from build123d import *

# Parameters (mm, degrees)
PAD002_DEPTH           = 18
CHAMFER001_SIZE        = 1
SKETCH004_W            = 20
SKETCH004_H            = 20
POCKET001_DEPTH        = 2
LINEARPATTERN001_COUNT = 3
LINEARPATTERN001_PITCH = 4
PAD003_DEPTH           = 6
CHAMFER002_SIZE        = 1


with BuildPart() as part:
    # Sketch003 → Pad002 (new body)
    with BuildSketch(Plane.XY):
        with BuildLine():
            ThreePointArc((8, 5.030159), (-9.45, 0), (8, -5.030159))
            Line((8, 5.030159), (8, -5.030159))
        make_face()
    extrude(amount=PAD002_DEPTH)

    # Chamfer001
    chamfer001_edges = [part.edges().sort_by_distance(p)[0] for p in [
        (-9.45, 0, 18),
        (8, 0, 18),
    ]]
    chamfer(chamfer001_edges, length=CHAMFER001_SIZE)

    # Sketch004 → Pocket001 (cut)
    with BuildSketch(Plane.XY.offset(3)):
        with Locations((12.12132, -12.12132)):
            Rectangle(SKETCH004_W, SKETCH004_H)
        with Locations((12.12132, 12.12132)):
            Rectangle(SKETCH004_W, SKETCH004_H)
        with Locations((-12.12132, 12.12132)):
            Rectangle(SKETCH004_W, SKETCH004_H)
        with Locations((-12.12132, -12.12132)):
            Rectangle(SKETCH004_W, SKETCH004_H)
    pocket001 = extrude(amount=POCKET001_DEPTH, mode=Mode.SUBTRACT)

    # LinearPattern001: Pocket001 ×3
    with Locations(*[(0, 0, i * LINEARPATTERN001_PITCH) for i in range(1, LINEARPATTERN001_COUNT)]):
        add(pocket001, mode=Mode.SUBTRACT)

    # Sketch005 → Pad003 (join)
    with BuildSketch(Plane.XY):
        Polygon((-12, 9), (-12, -13), (-11, -14), (7, -14), (8, -13), (8, 9), (7, 10), (-11, 10), align=None)
    extrude(amount=-PAD003_DEPTH)

    # Chamfer002
    chamfer002_edges = [part.edges().sort_by_distance(p)[0] for p in [
        (-2, 10, -6),
        (-11.5, 9.5, -6),
        (-12, -2, -6),
        (-11.5, -13.5, -6),
        (-2, -14, -6),
        (7.5, -13.5, -6),
        (8, -2, -6),
        (7.5, 9.5, -6),
    ]]
    chamfer(chamfer002_edges, length=CHAMFER002_SIZE)


solid = part.part
The listing builds one solid part. Answer for the finished solid, in the listing's coordinates (mm). A direction names the side the tool comes from. Give positions to 0.01 mm unless a question says otherwise; leave off trailing zeros. Write each loop counter-clockwise with the first axis right and the second up, starting at its lowest first coordinate (ties: lowest second). Pieces come first, ordered by that corner, then holes.
1) Section A-A (y = 0) is taken. Write down the section's boundary in (x, z), and give its area (3 significant figures).
2) Section B-B (x = 0) is taken. Write down the section's boundary in (y, z).
3) Find the intervals of material crossed by L1, parallel to Z at x = 3.5, y = 6; L2, parallel to Z at x = 7.25, y = -5.75; L3, parallel to Z at x = -1, y = -11.75, in increasing order.
4) For a pull along Z with two mould halves and no side action, classify faces 1 (the face through (-2, -2, -6)), 2 (the face through (-5, -5, 11)), 3 (the face through (-12, -2, -2)) as pulls with the +Z half, pulls with the -Z half, needs draft (parallel to the pull), parting line crosses it, or undercut.
5) Given P1, Ø12, axis at x = 4.5, z = 15, coming from the -Y side; P2, Ø2, axis at y = -6.5, z = 11.5, coming from the -X side; P3, Ø1, axis at x = -6.5, z = 12, coming from the -Y side, each flat-ended and moving along its own axis, determine where each tip first touches the part or whether it passes through.
6) A tool of negligible diameter and unlimited length cuts with its end or side. For faces 4 (the face through (4, -5, 7)), 5 (the face through (5, 2.121, 4)), 6 (the face through (-6, -2.121, 4)), from which of +Z, -Z, +X, -X, +Y, -Y can it reach the whole face along a straight path? Write none if from no direction.
7) Section C-C (z = 14.5) is taken. Write down the section's boundary in (x, y).
Response:
1. outline: (-12, -5) - (-11, -6) - (7, -6) - (8, -5) - (8, 17) - (7, 18) - (-8.45, 18) - (-9.45, 17) - (-9.45, 0) - (-12, 0) - close
1. area: 432 mm2
2. outline: (-14, -5) - (-13, -6) - (9, -6) - (10, -5) - (10, 0) - (9.45, 0) - (9.45, 17) - (8.45, 18) - (-8.45, 18) - (-9.45, 17) - (-9.45, 0) - (-14, 0) - close
3. L1: z = -6 to 3, 5 to 7, 9 to 11, 13 to 18
3. L2: z = -5.75 to 3, 5 to 7, 9 to 11, 13 to 17.2
3. L3: z = -6 to 0
4. face 1: pulls with the -Z half
4. face 2: undercut
4. face 3: needs draft
5. P1: stops at y = -9.45
5. P2: stops at x = -7.59
5. P3: stops at y = -2.12
6. face 4: +X, -Y
6. face 5: +X, +Y
6. face 6: -X, -Y
7. outline: (8, -5.03) - (8, 5.03) arc R9.45 ccw (long way) to start
